Build history of the part. All positions in model axes, mm. Face numbers are marked on the shaded views. A direction names the side the tool comes from. Round coordinates to 2 decimals unless told otherwise and drop trailing zeros. Write each loop counter-clockwise with the first axis right and the second up, starting at its lowest first coordinate (ties: lowest second). Pieces come first, ordered by that corner, then holes. Notation, with made-up numbers: M 51,13.5 L 107,13.5 A10 ccw 107,17.5 Z; hole C 23.5,51.25 d11. An arc over 180 degrees is marked long. Write item = value, one per line.
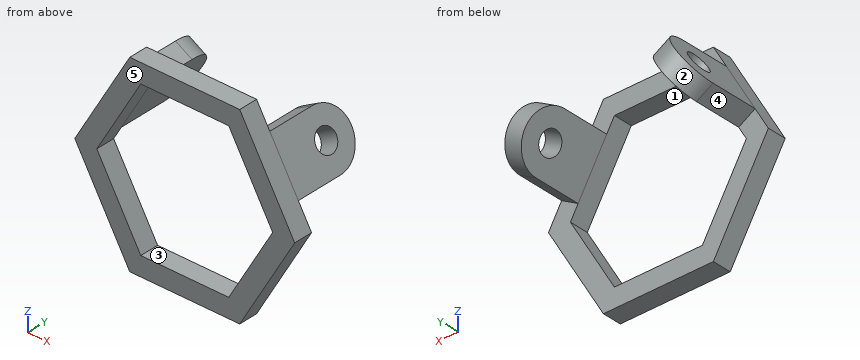
from build123d import *

# Parameters (mm, degrees)
BOSS_EXTRUDE1_DEPTH = 10
SKETCH2_R           = 6
BOSS_EXTRUDE2_DEPTH = 10


with BuildPart() as part:
    # Sketch1 → Boss-Extrude1 (new body)
    with BuildSketch(Plane(origin=(0, 0, 0), x_dir=(1, 0, 0), z_dir=(0, 1, 0))):
        Polygon((57.735026919, 0), (28.867513459, 50), (-28.867513459, 50), (-57.735026919, 0), (-28.867513459, -50), (28.867513459, -50), align=None)
        Polygon((23.094010768, 40), (-23.094010768, 40), (-46.188021535, 0), (-23.094010768, -40), (23.094010768, -40), (46.188021535, 0), align=None, mode=Mode.SUBTRACT)
    extrude(amount=BOSS_EXTRUDE1_DEPTH)

    # Sketch2 → Boss-Extrude2 (add)
    with BuildSketch(Plane(origin=(43.301270189, 0, 25), x_dir=(0.4999999999999951, 0, -0.8660254037844415), z_dir=(0.8660254037844416, 0, 0.49999999999999517))):
        with BuildLine():
            Line((-15, 35), (-15, 10))
            Line((-15, 10), (15, 10))
            Line((15, 10), (15, 35))
            ThreePointArc((15, 35), (0, 50), (-15, 35))
        make_face()
        with Locations((0, 35)):
            Circle(SKETCH2_R, mode=Mode.SUBTRACT)
    boss_extrude2 = extrude(amount=-BOSS_EXTRUDE2_DEPTH)

    # Mirror7: Boss-Extrude2 across plane
    add(boss_extrude2.mirror(Plane(origin=(0, 0, 0), x_dir=(0, 0, 1), z_dir=(1, 0, 0))))


solid = part.part
1. Mould opens along Z. For the marked faces 3, 4 and 5 say: pulls with the +Z half, pulls with the -Z half, needs draft (parallel to the pull), parting line crosses it, or undercut.
Responses:
face_3 = undercut
face_4 = pulls with the -Z half
face_5 = needs draft
2. Band-saw the part on D-D (y = 38). List the corners of the cut face in (x, z), plus the area to 3 significant figures.
Responses:
outline = M -50.65,12.27 L -41.99,7.27 L -37.24,15.5 L -45.9,20.5 Z; M -40.7,29.5 L -32.04,24.5 L -27.29,32.73 L -35.95,37.73 Z; M 27.29,32.73 L 32.04,24.5 L 40.7,29.5 L 35.95,37.73 Z; M 37.24,15.5 L 41.99,7.27 L 50.65,12.27 L 45.9,20.5 Z
area = 380 mm²
3. Flat gauge pins, fed straight in: pin 1 (1.5 mm diameter, centred on y = 16, z = 24.5, fed in from -X); pin 2 (6 mm diameter, centred on x = -37.5, z = 38, fed in from +Y); pin 3 (4 mm diameter, centred on x = -28, z = 32.5, fed in from +Y); pin 4 (6 mm diameter, centred on x = 20.5, y = 15, fed in from +Z). Where does each tip first touch, or does it go through?
Responses:
pin_1 = -44.02
pin_2 = 44.57
pin_3 = 43.8
pin_4 = through
4. Band-saw the part on B-B (x = -12.5). List the corners of the cut face in (y, z), plus the area to 3 significant figures.
Responses:
outline = M 0,-50 L 10,-50 L 10,-40 L 0,-40 Z; M 0,40 L 10,40 L 10,50 L 0,50 Z
area = 200 mm²
5. Tool access for the marked faces 1 and 2: list every direction of +Z, -Z, +X, -X, +Y, -Y with a clear straight run to the whole face (end or side of a thin tool).
Responses:
face_1 = +Y, -Y
face_2 = +Y
6. Probe probe 1 along Z at (x, y) = (16, 6); probe 2 along Y at (x, z) = (41, -27.5); probe 3 along X at (y, z) = (43.5, 28.5). List the from-to ranges inside material, lowest first.
Responses:
probe_1 = -50 to -40, 40 to 50
probe_2 = 0 to 10
probe_3 = -41.28 to -29.73, 29.73 to 41.28
7. Band-saw the part on A-A (y = 20.5). List the corners of the cut face in (x, z).
Responses:
outline = M -50.8,12.01 L -42.14,7.01 L -27.14,32.99 L -35.8,37.99 Z; M 27.14,32.99 L 42.14,7.01 L 50.8,12.01 L 35.8,37.99 Z
8. Band-saw the part on C-C (y = 7). List the corners of the cut face in (x, z).
Responses:
outline = M -57.74,0 L -28.87,-50 L 28.87,-50 L 57.74,0 L 28.87,50 L -28.87,50 Z; hole M -46.19,0 L -23.09,-40 L 23.09,-40 L 46.19,0 L 23.09,40 L -23.09,40 Z
